Read the model definition and answer for the solid it produces. Units are mm, in the model's axes. A direction names the side the tool comes from. Round coordinates to 2 decimals unless told otherwise and drop trailing zeros. Write each loop counter-clockwise with the first axis right and the second up, starting at its lowest first coordinate (ties: lowest second). Pieces come first, ordered by that corner, then holes. Notation, with made-up numbers: (19, 89) - (41, 89) arc R33 ccw to (41, 126) - close; hole circle Ø11 at (16.5, 41). An arc over 180 degrees is marked (long way). Answer as CSV lines item,"result". Start each with the question number.
1) Find section C-C on y = 14. Determine the outline of the cut face in (x, z).
2) Each of these flat-tipped pins is pushed along its axis until it touches: pin 1 (2 mm diameter, centred on x = 0, y = 29, fed in from +Z); pin 2 (0.6 mm diameter, centred on x = 4.5, y = 12.5, fed in from +Z); pin 3 (1.6 mm diameter, centred on x = 4.5, y = 7, fed in from -Z). Where does it stop, or does it pass through?
3) Find section D-D on z = 11. Determine the outline of the cut face in (x, y), then the cut area to 3 significant figures.
4) Find section B-B on z = 23. Determine the outline of the cut face in (x, y).
5) Consider line 1 along Z through (x, y) = (21.5, 3); line 2 along X through (y, z) = (26.5, 21); line 3 along X through (y, z) = (32.5, 22). Determine where each line is inside the solid, lowest interval first.
6) For a pull along X with two mould halves and no side action, classify faces 4 (the flat face through (4, 12, 18.571)), 5 (the flat face through (-16.545, 12, 26)), 6 (the flat face through (-14, 12, 8.571)) as +X half, -X half, draft (parallel to the pull), parting line (faces both ways), or undercut.
7) Find section A-A on x = 22. Determine the outline of the cut face in (y, z), then the cut area to 3 significant figures.
8) Which of the six approach directions +Z, -Z, +X, -X, +Y, -Y give full straight-line access (tool end or side, diameter ignored) to faces 1 (the flat face through (19.455, 12, 14)), 2 (the flat face through (-10.545, 12, 14)), 3 (the flat face through (12.85, 12.336, 25.966))?
from build123d import *

# Parameters (mm, degrees)
F1_DEPTH = 12


with BuildPart() as f1:
    # F0 (on Front) → F1 (new body, symmetric)
    with BuildSketch(Plane.XZ):
        Polygon((-16.544905, 8.570568), (-16.544905, -6.429432), (-6.544905, -6.429432), (3.455095, 3.570568), (4.455095, 3.570568), (4.455095, 18.570568), (3.455095, 18.570568), (-11.544905, 33.570568), (-16.544905, 33.570568), (-16.544905, 18.570568), (-10.544905, 18.570568), (-10.544905, 8.570568), align=None)
    extrude(amount=F1_DEPTH, both=True)

    # F2: F1 across face


with BuildPart() as f1_1:
    add(f1.part)
    add(f1.part.mirror(Plane(origin=(-7.082177, 12, 12.065645), x_dir=(1, 0, 0), z_dir=(0, 1, 0))))

    # F3: F1 across face


with BuildPart() as f1_2:
    add(f1_1.part)
    add(f1_1.part.mirror(Plane(origin=(4.455095, 12, 11.070568), x_dir=(0, 1, 0), z_dir=(1, 0, 0))))


solid = f1_2.part
Check values:
1,outline,"(-16.54, -6.43) - (-6.54, -6.43) - (3.46, 3.57) - (5.46, 3.57) - (15.46, -6.43) - (25.46, -6.43) - (25.46, 8.57) - (19.46, 8.57) - (19.46, 18.57) - (25.46, 18.57) - (25.46, 33.57) - (20.46, 33.57) - (5.46, 18.57) - (3.46, 18.57) - (-11.54, 33.57) - (-16.54, 33.57) - (-16.54, 18.57) - (-10.54, 18.57) - (-10.54, 8.57) - (-16.54, 8.57) - close"
2,pin 1,"stops at z = 23.03"
2,pin 2,"stops at z = 18.57"
2,pin 3,"stops at z = 3.57"
3,outline,"(-10.54, -12) - (19.46, -12) - (19.46, 36) - (-10.54, 36) - close"
3,area,"1,440 mm^2"
4,outline,"(-16.54, -12) - (-0.97, -12) - (-0.97, 36) - (-16.54, 36) - close; (9.88, -12) - (25.46, -12) - (25.46, 36) - (9.88, 36) - close"
5,line 1,"z = -6.43 to 8.57, 18.57 to 33.57"
5,line 2,"x = -16.54 to 1.03, 7.88 to 25.46"
5,line 3,"x = -16.54 to 0.03, 8.88 to 25.46"
6,face 4,"undercut"
6,face 5,"-X half"
6,face 6,"draft"
7,outline,"(-12, -6.43) - (36, -6.43) - (36, 8.57) - (-12, 8.57) - close; (-12, 18.57) - (36, 18.57) - (36, 33.57) - (-12, 33.57) - close"
7,area,"1,440 mm^2"
8,face 1,"+X, +Y, -Y"
8,face 2,"-X, +Y, -Y"
8,face 3,"+Z, +Y, -Y"
